Work out the finished part from the listing and answer in its coordinate system (mm). Face numbers are marked on the shaded views. A direction names the side the tool comes from. Round coordinates to 2 decimals unless told otherwise and drop trailing zeros. Loops run counter-clockwise (first coordinate to the right, second up) from the corner with the lowest first, then second, coordinate; pieces in that order, holes last.
```python
from build123d import *

# Parameters (mm, degrees)
F0_R     = 0.79375
F0_W     = 6.35
F0_H     = 25.4
F0_R_2   = 1.63195
F0_R_3   = 1.35255
F1_DEPTH = 6.35
F2_DEPTH = 5.08
F3_R     = 1.35255
F4_DEPTH = 6.35


with BuildPart() as f1:
    # F0 (on Top) → F1 (new body)
    with BuildSketch(Plane.XY):
        Polygon((-3.175, 25.146), (-3.175, 12.7), (3.175, 12.7), (3.175, 25.146), (3.175, 28.956), (-3.175, 28.956), align=None)
        with Locations((0, 25.146)):
            Circle(F0_R, mode=Mode.SUBTRACT)
        Rectangle(F0_W, F0_H)
        with Locations((0, -6.35)):
            Circle(F0_R_2, mode=Mode.SUBTRACT)
        with Locations((0, 5.08)):
            Circle(F0_R_3, mode=Mode.SUBTRACT)
        with Locations((0, 5.08)):
            Circle(F0_R_3)
    extrude(amount=F1_DEPTH)

    # F0 (on Top) → F2 (cut)
    with BuildSketch(Plane.XY):
        with Locations((0, 5.08)):
            Circle(F0_R_3)
    extrude(amount=F2_DEPTH, mode=Mode.SUBTRACT)

    # F3 (on face) → F4 (join)
    with BuildSketch(Plane.XZ.offset(12.7)):
        with Locations((0, 3.175)):
            Circle(F3_R)
    extrude(amount=F4_DEPTH)


solid = f1.part
```
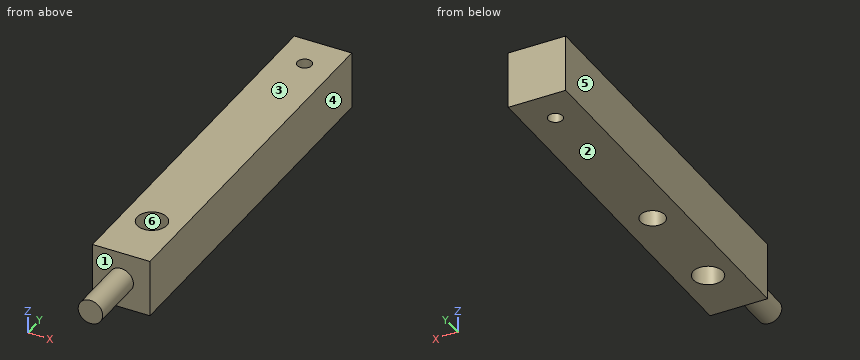
1. Determine the mould class of the marked faces 3, 4, 5 and 6 for opening direction X: +X half, -X half, draft (parallel to the pull), parting line (faces both ways), or undercut.
Answer key:
face 3: draft
face 4: +X half
face 5: -X half
face 6: undercut
2. Given pin 1 (1 mm diameter, centred on x = 0, y = 25.146, fed in from +Z), flat-ended and moving along its own axis, determine where the tip first touches the part or whether it passes through.
Answer key:
pin 1: passes through
3. Find section B-B (x = 0). Write down the section's boundary in (y, z), then the cut area to 3 significant figures.
Answer key:
outline: (-19.05, 1.82) - (-12.7, 1.82) - (-12.7, 0) - (-7.98, 0) - (-7.98, 6.35) - (-12.7, 6.35) - (-12.7, 4.53) - (-19.05, 4.53) - close; (-4.72, 0) - (3.73, 0) - (3.73, 5.08) - (6.43, 5.08) - (6.43, 0) - (24.35, 0) - (24.35, 6.35) - (-4.72, 6.35) - close; (25.94, 0) - (28.96, 0) - (28.96, 6.35) - (25.94, 6.35) - close
area: 237 mm2
4. Consider probe 1 along Y at (x, z) = (0, 2.25); probe 2 along X at (y, z) = (-6.5, 5) (3 decimals); probe 3 along Y at (x, z) = (0, 5). Determine where each line is inside the solid, lowest interval first.
Answer key:
probe 1: y = -19.05 to -7.98, -4.72 to 3.73, 6.43 to 24.35, 25.94 to 28.96
probe 2: x = -3.175 to -1.625, 1.625 to 3.175
probe 3: y = -12.7 to -7.98, -4.72 to 3.73, 6.43 to 24.35, 25.94 to 28.96
5. Find section A-A (y = -6.35). Write down the section's boundary in (x, z) (3 decimals), then the cut area to 3 significant figures.
Answer key:
outline: (-3.175, 0) - (-1.632, 0) - (-1.632, 6.35) - (-3.175, 6.35) - close; (1.632, 0) - (3.175, 0) - (3.175, 6.35) - (1.632, 6.35) - close
area: 19.6 mm2
6. Which of the six approach directions +Z, -Z, +X, -X, +Y, -Y give full straight-line access (tool end or side, diameter ignored) to the marked faces 1 and 2?
Answer key:
face 1: -Y
face 2: -Z, +X, -X, +Y, -Y
7. Find section D-D (x = 2.5). Write down the section's boundary in (y, z), then the cut area to 3 significant figures.
Answer key:
outline: (-12.7, 0) - (28.96, 0) - (28.96, 6.35) - (-12.7, 6.35) - close
area: 265 mm2
8. Find section C-C (y = 5.08). Write down the section's boundary in (x, z) (3 decimals).
Answer key:
outline: (-3.175, 0) - (-1.353, 0) - (-1.353, 5.08) - (1.353, 5.08) - (1.353, 0) - (3.175, 0) - (3.175, 6.35) - (-3.175, 6.35) - close
